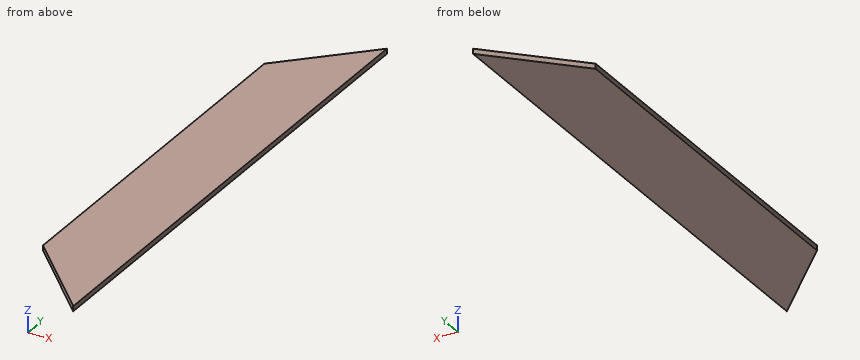
```python
from build123d import *

# Parameters (mm, degrees)
F0_W          = 150
F0_H          = 10
F1_DEPTH      = 1019
F3_DEPTH      = 10.001
F3_DEPTH_BACK = 1540
F5_DEPTH      = 1577
F5_DEPTH_BACK = 10.001


# Not quite as in the source:
# - an extrude ends at something that could not be found from the text; its depth is read off the source's solid


with BuildPart() as f1:
    # F0 (on Front) → F1 (new body)
    with BuildSketch(Plane.XZ):
        with Locations((0.4800241441, -31.7408985884)):
            Rectangle(F0_W, F0_H)
    extrude(amount=F1_DEPTH)

    # F2 (on face) → F3 (cut, two sides)
    with BuildSketch(Plane.XY.offset(-26.7408985884)) as f3_sk:
        Polygon((-74.5199758559, -150), (75.4800241441, 0), (178.0070960522, 169.0949052572), (-164.1357541084, 159.836769104), (-164.1357541084, -150), (-107.9861149192, -156.7480415106), align=None)
    extrude(amount=-F3_DEPTH, mode=Mode.SUBTRACT)
    extrude(f3_sk.sketch, amount=F3_DEPTH_BACK, mode=Mode.SUBTRACT)

    # F4 (on face) → F5 (cut, two sides)
    with BuildSketch(Plane.XY.offset(-26.7408985884)) as f5_sk:
        Polygon((72.7586299181, -1200.1620531082), (75.4800241441, -1019), (-74.5199758559, -869), (-237.236186862, -869), (-237.236186862, -1200.1620531082), align=None)
    extrude(amount=F5_DEPTH, mode=Mode.SUBTRACT)
    extrude(f5_sk.sketch, amount=-F5_DEPTH_BACK, mode=Mode.SUBTRACT)


solid = f1.part
```
Input: part model. Units: mm. Frame: model coordinates. Coordinates: 2 decimals unless noted, no trailing zeros. Loops run counter-clockwise (first coordinate to the right, second up) from the corner with the lowest first, then second, coordinate; pieces in that order, holes last.
Q1. Section A-A, the plane x = 0. Return the cut outline in (y, z).
Results are:
outline: (-943.52, -36.74) - (-75.48, -36.74) - (-75.48, -26.74) - (-943.52, -26.74) - close
Q2. Line query: line 1 along Y through (x, z) = (-51, -31.25); line 2 along Y through (x, z) = (-18.5, -33.5); line 3 along X through (y, z) = (-51, -28.75). Output: solid intervals per line, ascending.
Results are:
line 1: y = -892.52 to -126.48
line 2: y = -925.02 to -93.98
line 3: x = 24.48 to 75.48
Q3. Section B-B, the plane y = -128. Return the cut outline in (x, z).
Results are:
outline: (-52.52, -36.74) - (75.48, -36.74) - (75.48, -26.74) - (-52.52, -26.74) - close
